Geometry: final body of the model. Coordinates: model frame, mm. Face numbers are marked on the shaded views. A direction names the side the tool comes from. Round coordinates to 2 decimals unless told otherwise and drop trailing zeros. Order: outer loops, then holes, each group sorted by start corner. A loop starts at its lowest first (then second) coordinate and runs counter-clockwise, first axis right, second up. Notation, with made-up numbers: M -15.75,51.5 L -9.75,51.5 A20 ccw -9.75,74.5 Z; hole C 88,30 d3. An arc over 180 degrees is marked long. Put each result on its own line as item: value. Start each with the question number.
1) Section A-A, the plane z = 35.5. Return loops of the section in (x, y), then the cut area to 3 significant figures.
2) Section B-B, the plane y = 146. Return loops of the section in (x, z), then the cut area to 3 significant figures.
3) Section D-D, the plane z = -8.5. Return loops of the section in (x, y), then the cut area to 3 significant figures.
4) Section C-C, the plane x = -387. Return loops of the section in (y, z).
5) Access query for the marked faces 1 and 2. Directions: +Z, -Z, +X, -X, +Y, -Y. A direction counts if a zero-diameter tool reaches every point of the face in a straight line with its end or side. Return the directions, or none.
6) Material intervals for probe 1 along Y at (x, z) = (-291.5, 1.5) (3 decimals); probe 2 along X at (y, z) = (114, -13.5); probe 3 along Y at (x, z) = (445.5, 3), sorted ascending. Write a range as [from, to].
7) First-contact query: P1, Ø1.8, axis at y = -41.5, z = 12.5, coming from the +X side; P2, Ø10, axis at y = 127, z = -13, coming from the -X side; P3, Ø1.5, axis at x = 498, y = 42.5, coming from the -Z side. Flat tips, straight axial feed; report the tip coordinate or a pass-through.
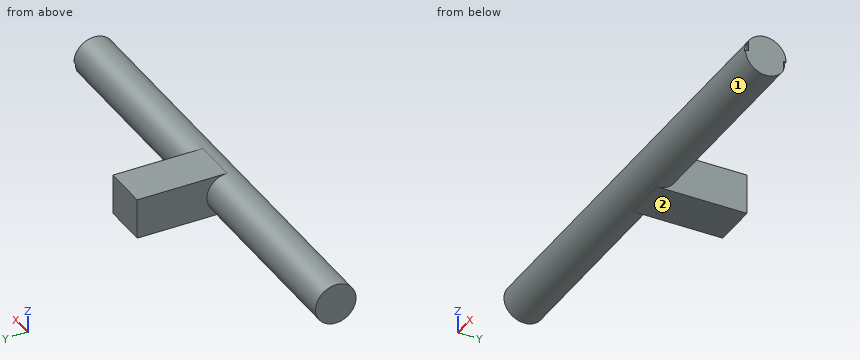
from build123d import *

# Parameters (mm, degrees)
ESQUISSE1_R             = 45
BOSS_EXTRU_1_DEPTH      = 500
ESQUISSE2_W             = 90
ESQUISSE2_H             = 200
BOSS_EXTRU_2_DEPTH      = 50
ESQUISSE7_W             = 22.449944321
ESQUISSE7_H             = 6
ENL_V_MAT_EXTRU_1_DEPTH = 5


with BuildPart() as part:
    # Esquisse1 → Boss.-Extru.1 (new body, symmetric)
    with BuildSketch(Plane(origin=(0, 0, 0), x_dir=(0, 0, -1), z_dir=(1, 0, 0))):
        Circle(ESQUISSE1_R)
    extrude(amount=BOSS_EXTRU_1_DEPTH, both=True)

    # Esquisse2 → Boss.-Extru.2 (add, symmetric)
    with BuildSketch(Plane(origin=(0, 0, 0), x_dir=(0, 0, -1), z_dir=(1, 0, 0))):
        with Locations((0, 100)):
            Rectangle(ESQUISSE2_W, ESQUISSE2_H)
    extrude(amount=BOSS_EXTRU_2_DEPTH, both=True)

    # Esquisse7 → Enlèv. mat.-Extru.1 (cut)
    with BuildSketch(Plane(origin=(500, 0, 0), x_dir=(0, 0, -1), z_dir=(1, 0, 0))):
        with Locations((11.224972161, 42)):
            Rectangle(ESQUISSE7_W, ESQUISSE7_H)
        with Locations((-11.224972161, -42)):
            Rectangle(ESQUISSE7_W, ESQUISSE7_H)
    extrude(amount=-ENL_V_MAT_EXTRU_1_DEPTH, mode=Mode.SUBTRACT)


solid = part.part
Result sheet:
1. outline: M -500,-27.65 L 500,-27.65 L 500,27.65 L 50,27.65 L 50,200 L -50,200 L -50,27.65 L -500,27.65 Z
1. area: 72,500 mm2
2. outline: M -50,-45 L 50,-45 L 50,45 L -50,45 Z
2. area: 9,000 mm2
3. outline: M -500,-44.19 L 500,-44.19 L 500,39 L 495,39 L 495,44.19 L 50,44.19 L 50,200 L -50,200 L -50,44.19 L -500,44.19 Z
3. area: 104,000 mm2
4. outline: C 0,0 d90
5. face 1: none
5. face 2: -Z, +X, -X, +Y, -Y
6. probe 1: y = [-44.975, 44.975]
6. probe 2: x = [-50, 50]
6. probe 3: y = [-44.9, 44.9]
7. P1: stops at x = 495
7. P2: stops at x = -50
7. P3: stops at z = 0
